Check sheet for the drawn part. Datum: minimum x, y, z corner. Units: mm. Round coordinates to 2 decimals unless told otherwise and drop trailing zeros. Write each loop counter-clockwise with the first axis right and the second up, starting at its lowest first coordinate (ties: lowest second). Pieces come first, ordered by that corner, then holes. Notation, with made-up numbers: (-12.75, 63.5) - (30.25, 63.5) arc R26 cw to (30.25, 87.5) - close; hole circle Ø9 at (80.5, -19). An arc over 180 degrees is marked (long way). Write each question's results on one line, items separated by ' | '.
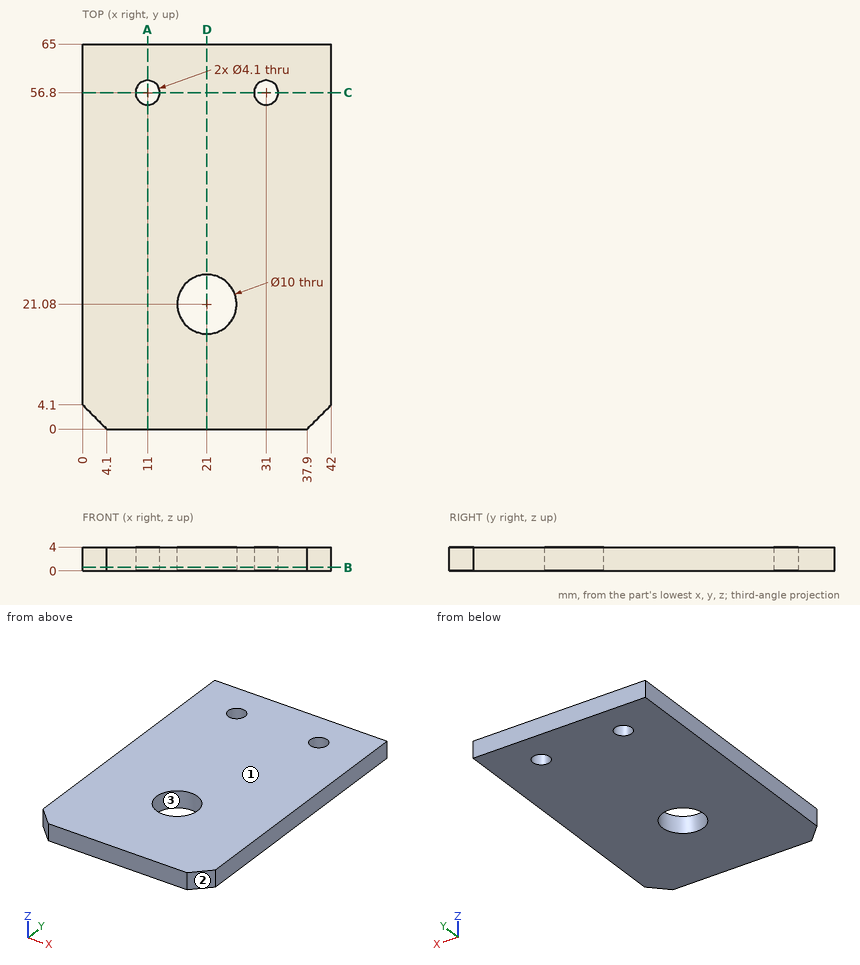
(1) Mould release check, pull along X, two halves, no side actions. Record for the marked faces 1, 2 and 3: released by +X, released by -X, zero draft, split by the parting line, or undercut.
Answer:
face 1: zero draft | face 2: released by +X | face 3: undercut
(2) Section check B-B (z = 0.6). Record the cut outline in (x, y), plus the area to 3 significant figures.
Answer:
outline: (0, 4.1) - (4.1, 0) - (37.9, 0) - (42, 4.1) - (42, 65) - (0, 65) - close; hole circle Ø4.1 at (11, 56.8); hole circle Ø10 at (21, 21.08); hole circle Ø4.1 at (31, 56.8) | area: 2,610 mm2
(3) Thickness scan on L1, parallel to Y at x = 11, z = 1.4; L2, parallel to X at y = 56.5, z = 2.5; L3, parallel to Y at x = 21, z = 2.55. Record the ranges inside material, lowest first.
Answer:
L1: 0 to 54.75, 58.85 to 65 | L2: 0 to 8.97, 13.03 to 28.97, 33.03 to 42 | L3: 0 to 16.08, 26.08 to 65
(4) Section check D-D (x = 21). Record the cut outline in (y, z).
Answer:
outline: (0, 0) - (16.08, 0) - (16.08, 4) - (0, 4) - close; (26.08, 0) - (65, 0) - (65, 4) - (26.08, 4) - close
(5) Section check A-A (x = 11). Record the cut outline in (y, z).
Answer:
outline: (0, 0) - (54.75, 0) - (54.75, 4) - (0, 4) - close; (58.85, 0) - (65, 0) - (65, 4) - (58.85, 4) - close
(6) Section check C-C (y = 56.8). Record the cut outline in (x, z), plus the area to 3 significant figures.
Answer:
outline: (0, 0) - (8.95, 0) - (8.95, 4) - (0, 4) - close; (13.05, 0) - (28.95, 0) - (28.95, 4) - (13.05, 4) - close; (33.05, 0) - (42, 0) - (42, 4) - (33.05, 4) - close | area: 135 mm2
